from build123d import *

# Parameters (mm, degrees)
F0_R     = 1.5
F1_DEPTH = 7
F3_DEPTH = 2
F4_R     = 1.5
F5_DEPTH = 1.5
F6_R     = 1.49999


# Not quite as in the source:
# - a fillet or chamfer is up to 0.001 mm smaller than in the source, because OpenCascade refuses the exact size


with BuildPart() as f1:
    # F0 (on Front) → F1 (new body)
    with BuildSketch(Plane.XZ):
        Circle(F0_R)
    extrude(amount=F1_DEPTH)

    # F2 (on face) → F3 (join)
    with BuildSketch(Plane.XZ.offset(7)):
        with BuildLine():
            ThreePointArc((1.2976046011, -0.752477441), (1.4485176736, -0.3896107662), (1.5, 0))
            ThreePointArc((1.5, 0), (1.4485176736, 0.3896107662), (1.2976046011, 0.752477441))
            Line((1.2976046011, 0.752477441), (-1.2976046011, 0.752477441))
            ThreePointArc((-1.2976046011, 0.752477441), (-1.5, 0), (-1.2976046011, -0.752477441))
            Line((-1.2976046011, -0.752477441), (1.2976046011, -0.752477441))
        make_face()
        with BuildLine():
            ThreePointArc((1.2976046011, 0.752477441), (1.4485176736, 0.3896107662), (1.5, 0))
            ThreePointArc((1.5, 0), (1.4485176736, -0.3896107662), (1.2976046011, -0.752477441))
            Line((1.2976046011, -0.752477441), (3.9969966747, -0.752477441))
            Line((3.9969966747, -0.752477441), (3.9969966747, 0.752477441))
            Line((3.9969966747, 0.752477441), (1.2976046011, 0.752477441))
        make_face()
        with BuildLine():
            Line((-1.2976046011, 0.752477441), (1.2976046011, 0.752477441))
            ThreePointArc((1.2976046011, 0.752477441), (0, 1.5), (-1.2976046011, 0.752477441))
        make_face()
        with BuildLine():
            ThreePointArc((-1.2976046011, -0.752477441), (0, -1.5), (1.2976046011, -0.752477441))
            Line((1.2976046011, -0.752477441), (-1.2976046011, -0.752477441))
        make_face()
        with BuildLine():
            ThreePointArc((-1.2976046011, -0.752477441), (-1.5, 0), (-1.2976046011, 0.752477441))
            Line((-1.2976046011, 0.752477441), (-3.9969966747, 0.752477441))
            Line((-3.9969966747, 0.752477441), (-3.9969966747, -0.752477441))
            Line((-3.9969966747, -0.752477441), (-1.2976046011, -0.752477441))
        make_face()
    extrude(amount=F3_DEPTH)

    # F4 (on face) → F5 (join)
    with BuildSketch(Plane.XZ.offset(9)):
        Circle(F4_R)
    extrude(amount=F5_DEPTH)

    # F6 (radius 1.5 in the source; OpenCascade refuses exactly that, so slightly less here)
    f6_edges = [f1.edges().sort_by_distance(p)[0] for p in [
        (-1.5, -10.5, 0),
    ]]
    fillet(f6_edges, radius=F6_R)


solid = f1.part
Build history of the part. All positions in model axes, mm. A direction names the side the tool comes from. Round coordinates to 2 decimals unless told otherwise and drop trailing zeros. Write each loop counter-clockwise with the first axis right and the second up, starting at its lowest first coordinate (ties: lowest second). Pieces come first, ordered by that corner, then holes. Notation, with made-up numbers: M -9.75,-28 L 24.25,-28 A9 ccw 24.25,-21 Z; hole C -24.5,1 d7. An arc over 180 degrees is marked long. Use CSV: the item, a comma, the result in double quotes.
1. Saw through at B-B (x = -2.25). Give the cut face in (y, z).
Reply:
outline,"M -9,-0.75 L -7,-0.75 L -7,0.75 L -9,0.75 Z"
2. Saw through at A-A (y = -2). Give the cut face in (x, z).
Reply:
outline,"C 0,0 d3"
3. Flat gauge pins, fed straight in: pin 1 (2 mm diameter, centred on x = -2.5, y = -8, fed in from -Z); pin 2 (0.5 mm diameter, centred on x = -3, z = 0, fed in from -Y); pin 3 (1 mm diameter, centred on x = -3, y = -7.5, fed in from +Z). Where does each tip first touch, or does it go through?
Reply:
pin 1,"stops at z = -0.75"
pin 2,"stops at y = -9"
pin 3,"stops at z = 0.75"
4. Tool access for faces 1 (the face through (3, -8, -0.752)), 2 (the face through (3, -8, 0.752)), 3 (the face through (-3, -8, -0.752)), 4 (the face through (-3, -8, 0.752)): list every direction of +Z, -Z, +X, -X, +Y, -Y with a clear straight run to the whole face (end or side of a thin tool).
Reply:
face 1,"-Z, +X, +Y, -Y"
face 2,"+Z, +X, +Y, -Y"
face 3,"-Z, -X, +Y, -Y"
face 4,"+Z, -X, +Y, -Y"
5. Wall check: probe 1 along Z at (x, y) = (1.5, -8.5); probe 2 along X at (y, z) = (-5, -0.05); probe 3 along Z at (x, y) = (0.75, -5.25). Give the ranges that are in metal, low to high. Write a range as from..to.
Reply:
probe 1,"z = -0.75..0.75"
probe 2,"x = -1.5..1.5"
probe 3,"z = -1.3..1.3"
